The listing builds one solid part. Answer for the finished solid, in the listing's coordinates (mm). A direction names the side the tool comes from. Round coordinates to 2 decimals unless told otherwise and drop trailing zeros. Loops run counter-clockwise (first coordinate to the right, second up) from the corner with the lowest first, then second, coordinate; pieces in that order, holes last. Notation, with made-up numbers: (39, 76.25) -> (61, 76.25) arc R12 cw to (61, 90.25) -> close; hole circle Ø7 at (5, -2). An arc over 180 degrees is marked (long way). One line per question, with ' | ' between items.
from build123d import *

# Parameters (mm, degrees)
F1_DEPTH = 18


with BuildPart() as f1:
    # F0 (on Right) → F1 (new body)
    with BuildSketch(Plane.YZ):
        with BuildLine():
            Line((396.25, -115), (396.25, 115))
            Line((396.25, 115), (212.359541, 115))
            ThreePointArc((212.359541, 115), (197.026206, 112.590849), (183.170485, 105.595555))
            Line((183.170485, 105.595555), (128.138406, 66.026335))
            ThreePointArc((128.138406, 66.026335), (114.282684, 59.031041), (98.94935, 56.621889))
            Line((98.94935, 56.621889), (-98.94935, 56.621889))
            ThreePointArc((-98.94935, 56.621889), (-114.282684, 59.031041), (-128.138406, 66.026335))
            Line((-128.138406, 66.026335), (-183.170485, 105.595555))
            ThreePointArc((-183.170485, 105.595555), (-197.026206, 112.590849), (-212.359541, 115))
            Line((-212.359541, 115), (-396.25, 115))
            Line((-396.25, 115), (-396.25, -115))
            Line((-396.25, -115), (396.25, -115))
        make_face()
    extrude(amount=F1_DEPTH)


solid = f1.part
Q1. For faces 4 (the face through (9, -303, 115)), 5 (the face through (9, 1, 56.622)), determine the directions among +Z, -Z, +X, -X, +Y, -Y from which every point of the face is accessible in a straight line to the end or side of a thin tool.
Numbers:
face 4: +Z, +X, -X, +Y, -Y | face 5: +Z, +X, -X
Q2. Given pin 1 Ø1.5 at (x, y) = (9, 79) entering from +Z, flat-ended and moving along its own axis, determine where the tip first touches the part or whether it passes through.
Numbers:
pin 1: z = 56.62
Q3. For a pull along Y with two mould halves and no side action, classify faces 1 (the face through (9, -396.25, 2)), 2 (the face through (8.874, 197.234, 112.657)), 3 (the face through (9, -6, -115)) as pulls with the +Y half, pulls with the -Y half, needs draft (parallel to the pull), parting line crosses it, or undercut.
Numbers:
face 1: pulls with the -Y half | face 2: undercut | face 3: needs draft
Q4. Find the intervals of material crossed by line 1 (Z direction, x = 13.5, y = 89.5); line 2 (Y direction, x = 11.25, z = 93); line 3 (Z direction, x = 13.5, y = 202.5), in increasing order. Write a range as from..to.
Numbers:
line 1: -115..56.62 | line 2: -396.25..-165.65, 165.65..396.25 | line 3: -115..114.02
Q5. A cutting plane is placed at C-C on y = -135. Give the vertices of the cut face in (x, z).
Numbers:
outline: (0, -115) -> (18, -115) -> (18, 70.96) -> (0, 70.96) -> close
Q6. A cutting plane is placed at A-A on x = 6.75. Give the vertices of the cut face in (y, z), plus the area to 3 significant figures.
Numbers:
outline: (-396.25, -115) -> (396.25, -115) -> (396.25, 115) -> (212.36, 115) arc R50 ccw to (183.17, 105.6) -> (128.14, 66.03) arc R50 cw to (98.95, 56.62) -> (-98.95, 56.62) arc R50 cw to (-128.14, 66.03) -> (-183.17, 105.6) arc R50 ccw to (-212.36, 115) -> (-396.25, 115) -> close | area: 164,000 mm^2
Q7. A cutting plane is placed at B-B on y = -24. Give the vertices of the cut face in (x, z).
Numbers:
outline: (0, -115) -> (18, -115) -> (18, 56.62) -> (0, 56.62) -> close
